Design review of the part built by this model. Coordinates are the model's own, in mm. Coordinates: 2 decimals unless noted, no trailing zeros. Write each loop counter-clockwise with the first axis right and the second up, starting at its lowest first coordinate (ties: lowest second). Pieces come first, ordered by that corner, then holes.
Q1. Take a section at A-A, the plane x = -13. Write out the cut boundary in (y, z), plus the area to 3 significant figures.
Q2. For L1, parallel to Y at x = 70, z = 0.8; L2, parallel to Y at x = -14.5, z = 0.4; L3, parallel to X at y = -10, z = 1.75, list the stretches that pass through material, from the lowest coordinate up.
Q3. Take a section at C-C, the plane z = 2.1. State how many separate pieces and enclosed holes the cut face has, plus the area to 3 significant figures.
Q4. Take a section at B-B, the plane y = 1.5. Write out the cut boundary in (x, z).
Q5. For pin 1 Ø1.5 at (y, z) = (105, 1.5) entering from -X, flat-tipped, find the tip position at first contact; note if it passes through.
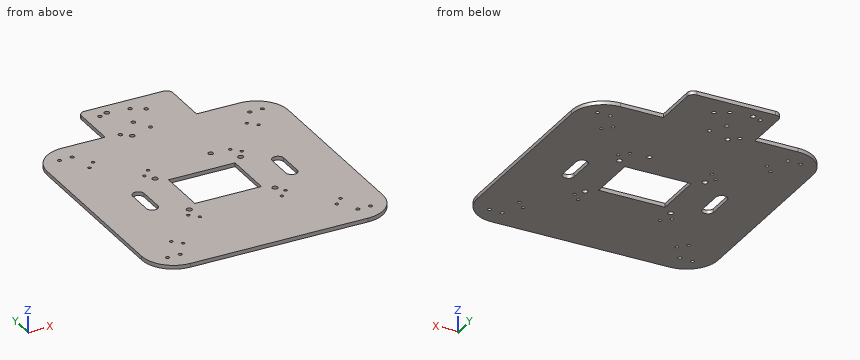
Autodesk Inventor part; units mm, degrees
ref_plane "YZ Plane" through (0, 0, 0) normal (1, 0, 0) x (0, 1, 0)
ref_plane "XZ Plane" through (0, 0, 0) normal (0, 1, 0) x (-1, 0, 0)
ref_plane "XY Plane" through (0, 0, 0) normal (0, 0, 1) x (1, 0, 0)
sketch "Sketch1" plane through (0, 0, 0) normal (0, 0, 1) x (1, 0, 0)
  point P0 (0, 0)
sketch "Sketch2" plane through (0, 0, 0) normal (0, 0, 1) x (1, 0, 0)
  line L0 (94.9998, -95.0001) -> (-94.9998, -95.0001)
  line L1 (-94.9998, -95.0001) -> (-94.9998, 95.0001)
  line L2 (-94.9998, 95.0001) -> (94.9998, 95.0001)
  line L3 (94.9998, 95.0001) -> (94.9998, -95.0001)
  line L4 (94.9998, -95.0001) -> (-94.9998, 95.0001) construction
  line L5 (-94.9998, -95.0001) -> (94.9998, 95.0001) construction
  line L6 (-36.0001, 94.9999) -> (36.0001, 94.9999)
  line L7 (36.0001, 94.9999) -> (36.0001, 135.0001)
  line L8 (36.0001, 135.0001) -> (-36.0001, 135.0001)
  line L9 (-36.0001, 135.0001) -> (-36.0001, 94.9999)
  line L10 (-36.0001, 94.9999) -> (36.0001, 135.0001) construction
  line L11 (36.0001, 94.9999) -> (-36.0001, 135.0001) construction
  point P0 (0, 115)
  point P1 (-36.0001, 95.0001)
  point P2 (36.0001, 95.0001)
extrude "Extrusion1" add sketch "Sketch2" along normal blind 3
sketch "Standoff holes" plane through (0, 0, 3) normal (0, 0, 1) x (1, 0, 0)
  circle A0 centre (70, 80) radius 1.5001
  circle A1 centre (70, -80) radius 1.5001
  circle A2 centre (-70, 80) radius 1.5001
  circle A3 centre (-70, -80) radius 1.5001
extrude "Extrusion2" cut sketch "Standoff holes" against normal blind 3
fillet "Fillet5" radius 25 4 edges at (-94.9998, 95.0001, 1.5) (94.9998, 95.0001, 1.5) (-94.9998, -95.0001, 1.5) (94.9998, -95.0001, 1.5)
fillet "Fillet6" radius 5 2 edges at (-36.0001, 135.0001, 1.5) (36.0001, 135.0001, 1.5)
sketch "Large Hammond mount holes" plane through (0, 0, 3) normal (0, 0, 1) x (1, 0, 0)
  circle A0 centre (17.6939, 39.717) radius 2.0002
  circle A1 centre (-18.3061, 125.717) radius 2.0002
  circle A2 centre (-18.3061, 87.967) radius 2.0002
sketch "PX4FLOW mount holes" plane through (0, 0, 0) normal (0, 0, -1) x (-1, 0, 0)
  circle A0 centre (25.0336, 123.3517) radius 1.5872
  circle A1 centre (1.2211, 123.3517) radius 1.5872
  circle A2 centre (1.2211, 123.3517) radius 1.5872
  circle A3 centre (1.2211, 93.1892) radius 1.5872
  circle A4 centre (25.0336, 93.1892) radius 1.5872
sketch "Guard rails mount holes" plane through (0, 0, 0) normal (0, 0, -1) x (-1, 0, 0)
  circle A0 centre (-32.3501, 38.3605) radius 1.2501
  circle A1 centre (-38.3605, 32.3501) radius 1.2501
  circle A2 centre (-60.6344, 66.6448) radius 1.2501
  circle A3 centre (-66.6448, 60.6344) radius 1.2501
  circle A4 centre (-38.3605, -32.3501) radius 1.2501
  circle A5 centre (-32.3501, -38.3605) radius 1.2501
  circle A6 centre (-66.6448, -60.6344) radius 1.2501
  circle A7 centre (-60.6344, -66.6448) radius 1.2501
  circle A8 centre (32.3501, -38.3605) radius 1.2501
  circle A9 centre (38.3605, -32.3501) radius 1.2501
  circle A10 centre (60.6344, -66.6448) radius 1.2501
  circle A11 centre (66.6448, -60.6344) radius 1.2501
  circle A12 centre (38.3605, 32.3501) radius 1.2501
  circle A13 centre (32.3501, 38.3605) radius 1.2501
  circle A14 centre (66.6448, 60.6344) radius 1.2501
  circle A15 centre (60.6344, 66.6448) radius 1.2501
sketch "Imperial standoffs" plane through (0, 0, 0) normal (0, 0, -1) x (-1, 0, 0)
  circle A0 centre (80, 80) radius 1.43
  circle A1 centre (-80, 80) radius 1.43
  circle A2 centre (-80, -80) radius 1.43
  circle A3 centre (80, -80) radius 1.43
extrude "Extrusion4" cut sketch "Large Hammond mount holes" against normal blind 10
extrude "Extrusion5" cut sketch "PX4FLOW mount holes" against normal blind 10
extrude "Extrusion6" cut sketch "Guard rails mount holes" against normal blind 10
extrude "Extrusion7" cut sketch "Imperial standoffs" against normal blind 10
sketch "Dual pol balun cutout" plane through (0, 0, 3) normal (0, 0, 1) x (1, 0, 0)
  line L0 (26.2, -19.4999) -> (-26.2, -19.4999)
  line L1 (-26.2, -19.4999) -> (-26.2, 19.4999)
  line L2 (-26.2, 19.4999) -> (26.2, 19.4999)
  line L3 (26.2, 19.4999) -> (26.2, -19.4999)
  line L4 (26.2, -19.4999) -> (-26.2, 19.4999) construction
  line L5 (-26.2, -19.4999) -> (26.2, 19.4999) construction
  point P0 (0, 0)
extrude "Extrusion8" cut sketch "Dual pol balun cutout" against normal blind 10
sketch "SONAR_holes" plane through (0, 0, 3) normal (0, 0, 1) x (1, 0, 0)
  circle A0 centre (-8.501, 105) radius 1.6502
  circle A1 centre (8.519, 117.95) radius 1.6502
extrude "Extrusion9" cut sketch "SONAR_holes" against normal blind 10
sketch "SONAR cutouts" plane through (0, 0, 3) normal (0, 0, 1) x (1, 0, 0)
  line L0 (-55.0003, -9.9996) -> (-55.0003, 9.9996) construction
  line L1 (-50.5008, -9.9996) -> (-50.5008, 9.9996)
  line L2 (-59.4997, 9.9996) -> (-59.4997, -9.9996)
  arc A0 (-59.4997, -9.9996) -> (-50.5008, -9.9996) centre (-55.0003, -9.9996) ccw
  arc A1 (-50.5008, 9.9996) -> (-59.4997, 9.9996) centre (-55.0003, 9.9996) ccw
  line L3 (54.9997, -9.9996) -> (54.9997, 9.9996) construction
  line L4 (59.4992, -9.9996) -> (59.4992, 9.9996)
  line L5 (50.5003, 9.9996) -> (50.5003, -9.9996)
  arc A2 (50.5003, -9.9996) -> (59.4992, -9.9996) centre (54.9997, -9.9996) ccw
  arc A3 (59.4992, 9.9996) -> (50.5003, 9.9996) centre (54.9997, 9.9996) ccw
  point P0 (0, 0)
  point P1 (-55.0003, 0)
  point P2 (54.9997, 0)
extrude "Extrusion10" cut sketch "SONAR cutouts" against normal blind 10
sketch "balun_support_holes" plane through (0, 0, 3) normal (0, 0, 1) x (1, 0, 0)
  circle A0 centre (0, 0) radius 2.1826
  circle A1 centre (33.74, 25.4) radius 2.1826
  circle A2 centre (33.74, -25.4) radius 2.1826
  circle A3 centre (-33.74, -25.4) radius 2.1826
  circle A4 centre (-33.74, 25.4) radius 2.1826
extrude "Extrusion13" cut sketch "balun_support_holes" against normal blind 10 contours A1 | A2 | A3 | A4
properties part number "payload_bay_square_dual_pol_balun" material "CFRP"
Responses:
1. outline: (-95, 0) - (-19.5, 0) - (-19.5, 3) - (-95, 3) - close; (19.5, 0) - (135, 0) - (135, 3) - (19.5, 3) - close
1. area: 573 mm2
2. L1: y = -95 to -81.5, -78.5 to 78.5, 81.5 to 95
2. L2: y = -95 to -19.5, 19.5 to 135
2. L3: x = -95 to -59.5, -50.5 to -26.2, 26.2 to 50.5, 59.5 to 95
3. separate pieces: 1
3. enclosed holes: 40
3. area: 35,600 mm2
4. outline: (-95, 0) - (-59.5, 0) - (-59.5, 3) - (-95, 3) - close; (-50.5, 0) - (-26.2, 0) - (-26.2, 3) - (-50.5, 3) - close; (26.2, 0) - (50.5, 0) - (50.5, 3) - (26.2, 3) - close; (59.5, 0) - (95, 0) - (95, 3) - (59.5, 3) - close
5. pin 1: stops at x = -36
